Work out the finished part from the listing and answer in its coordinate system (mm). Give positions to 0.01 mm unless a question says otherwise; leave off trailing zeros. Loops run counter-clockwise (first coordinate to the right, second up) from the corner with the lowest first, then second, coordinate; pieces in that order, holes last. Notation, with made-up numbers: (47.25, 49) - (62.25, 49) arc R30 ccw to (62.25, 82) - close; hole circle Ø5 at (-26, -17). An arc over 180 degrees is marked (long way). Use CSV: the item, a comma, the result in double quotes.
Autodesk Inventor part; units mm, degrees
ref_plane "YZ Plane" through (0, 0, 0) normal (1, 0, 0) x (0, 1, 0)
ref_plane "XZ Plane" through (0, 0, 0) normal (0, 1, 0) x (-1, 0, 0)
ref_plane "XY Plane" through (0, 0, 0) normal (0, 0, 1) x (1, 0, 0)
sketch "Sketch6" plane through (0, 0, 0) normal (0, 1, 0) x (-1, 0, 0)
  line L0 (0, 0) -> (-60.1073, 0)
  line L1 (-60.1073, 0) -> (-60.1073, 2980)
  line L2 (-60.1073, 2980) -> (0, 2980)
  line L3 (0, 2980) -> (0, 0)
  dimension "d26" = 60.1073
  dimension "d27" = 2980
extrude "Plate4" add sketch "Sketch6" along normal blind 3
sketch "Sketch9" plane through (0, 3, 0) normal (0, 1, 0) x (1, 0, 0)
  line L0 (0, -2980) -> (0, 0)
  line L1 (60.1073, -2980) -> (0, -2980)
  line L2 (60.1073, 0) -> (60.1073, -2980)
  line L3 (0, 0) -> (60.1073, 0)
  line L4 (25, -210) -> (10, -210) construction
  line L5 (10, -210) -> (10, -10) construction
  line L6 (10, -10) -> (25, -10) construction
  line L7 (25, -10) -> (25, -210) construction
  dimension "d44" = 200
  dimension "d45" = 15
  dimension "d46" = 10
  dimension "d47" = 10
sketch "Sketch7" plane through (0, 0, 0) normal (0, -1, 0) x (1, 0, 0)
  line L0 (0, 2980) -> (60.1073, 2980)
  line L1 (0, 0) -> (0, 2980)
  line L2 (60.1073, 0) -> (0, 0)
  line L3 (60.1073, 2980) -> (60.1073, 0)
  line L4 (0, 430.2) -> (31.0536, 430.2)
  line L5 (31.0536, 430.2) -> (31.0536, 427)
  line L6 (31.0536, 427) -> (0, 427)
  line L7 (0, 427) -> (0, 430.2)
  point P0 (0, 427)
  point P1 (0, 200)
  point P2 (46.4173, 200)
  point P3 (0, 427)
  dimension "d29" = 31.0536
  dimension "d30" = 3.2
  dimension "d31" = 427
extrude "Extrusion2" cut sketch "Sketch7" against normal through all contours L4 L5 L6 L1
pattern_linear "Rectangular Pattern1" count 5 spacing 500 along (0, 0, 1) of "Extrusion2"
sketch "Sketch8" plane through (0, 0, 0) normal (0, -1, 0) x (1, 0, 0)
  line L0 (0, 1930.2) -> (0, 2427)
  line L1 (0, 430.2) -> (31.0536, 430.2)
  line L2 (31.0536, 430.2) -> (31.0536, 427)
  line L3 (31.0536, 427) -> (0, 427)
  line L4 (0, 0) -> (0, 427)
  line L5 (60.1073, 0) -> (0, 0)
  line L6 (60.1073, 2980) -> (60.1073, 0)
  line L7 (0, 2980) -> (60.1073, 2980)
  circle A0 centre (0, 1490) radius 25
  line L8 (0, 1930.2) -> (31.0536, 1930.2)
  line L9 (31.0536, 1930.2) -> (31.0536, 1927)
  line L10 (31.0536, 1927) -> (0, 1927)
  line L11 (0, 1430.2) -> (0, 1927)
  line L12 (0, 1430.2) -> (31.0536, 1430.2)
  line L13 (31.0536, 1430.2) -> (31.0536, 1427)
  line L14 (31.0536, 1427) -> (0, 1427)
  line L15 (0, 930.2) -> (0, 1427)
  line L16 (0, 930.2) -> (31.0536, 930.2)
  line L17 (31.0536, 930.2) -> (31.0536, 927)
  line L18 (31.0536, 927) -> (0, 927)
  line L19 (0, 430.2) -> (0, 927)
  line L20 (0, 2430.2) -> (31.0536, 2430.2)
  line L21 (31.0536, 2430.2) -> (31.0536, 2427)
  line L22 (31.0536, 2427) -> (0, 2427)
  line L23 (0, 2430.2) -> (0, 2980)
  dimension "d37" = 50
  dimension "d38" = 1490
extrude "Extrusion3" cut sketch "Sketch8" against normal through all contours L11 A0 | A0 L11
pattern_linear "Rectangular Pattern2" count 3 spacing 1480 along (0, 0, 1) of "Extrusion3" first direction both ways yes
mark "Mark1"
chamfer "Corner Chamfer1" distance 6 angle 45 1 edges at (60.1073, 1.5, 2980)
equation "\"d26\" = Stringer4_deep"
equation "\"d28\" = Thickness"
equation "\"BendReliefWidth\" = Thickness"
equation "\"BendReliefDepth\" = 0.5 * Thickness"
equation "\"CornerReliefSize\" = 4 * Thickness"
equation "\"MinimumRemnant\" = 2 * Thickness"
equation "\"TransitionRadius\" = BendRadius"
equation "\"JacobiRadiusSize\" = BendRadius"
equation "\"GapSize\" = Thickness"
properties part number "BSH 0442 stringer 42" material "09g2s"
Item 1: Given P1, Ø0.9, axis at x = 10, y = 2, coming from the +Z side; P2, Ø0.9, axis at x = 23, y = 1, coming from the -Z side; P3, Ø0.9, axis at x = 18.5, y = 2, coming from the -Z side; P4, Ø1.5, axis at y = 1.5, z = 928.5, coming from the -X side, each flat-ended and moving along its own axis, determine where each tip first touches the part or whether it passes through.
Determined:
P1,"stops at z = 2947.29"
P2,"stops at z = 0"
P3,"stops at z = 26.31"
P4,"stops at x = 31.05"
Item 2: A cutting plane is placed at B-B on z = 1490. Determine the outline of the cut face in (x, y).
Determined:
outline,"(25, 0) - (60.11, 0) - (60.11, 3) - (25, 3) - close"
Item 3: Find the intervals of material crossed by line 1 (Z direction, x = 57.5, y = 2.75), in increasing order.
Determined:
line 1,"z = 0 to 2976.61"
